Source: CAD feature listing. Evaluate the final solid. Frame: model axes, mm. Face numbers are marked on the shaded views. A direction names the side the tool comes from. Round coordinates to 2 decimals unless told otherwise and drop trailing zeros. Order: outer loops, then holes, each group sorted by start corner. A loop starts at its lowest first (then second) coordinate and runs counter-clockwise, first axis right, second up. Notation, with made-up numbers: (10.25, 52) - (53.25, 52) arc R8 ccw to (53.25, 62) - close; hole circle Ø1 at (-25.5, 9.25). An arc over 180 degrees is marked (long way). Use one line per item in the form item = value. Start each with the question number.
Q1. Ray query, line 1 (Y direction, x = 28, z = -6.5); line 2 (Y direction, x = 25.5, z = -3.75); line 3 (X direction, y = -16, z = -9). Return the intervals inside material, ascending. Write a range as [from, to].
Q2. Pin query (flat end, axial travel): pin 1 Ø1.5 at (x, z) = (26, -7) entering from +Y; pin 2 Ø4 at (x, z) = (-2.5, -6.5) entering from +Y; pin 3 Ø13.5 at (x, y) = (0, 0) entering from -Z. Return the tip coordinate at first contact, or that it passes through.
Q3. Cut plane C-C, the plane y = 19. Return the cut outline in (x, z), and give its area (3 significant figures).
Q4. Draft query along Y for the marked faces 5, 6, 7 and 8. Return one class per face: released by +Y, released by -Y, zero draft, split by the parting line, or undercut.
Q5. Set-up query: the marked faces 1, 2, 3 and 4. Return all of +Z, -Z, +X, -X, +Y, -Y with unobstructed straight access to the full face (end or side cutting, diameter ignored); none if empty.
Q6. Cut plane A-A, the plane y = 6. Return the cut outline in (x, z), and give its area (3 significant figures).
Q7. Cut plane B-B, the plane y = -3. Return the cut outline in (x, z), and give its area (3 significant figures).
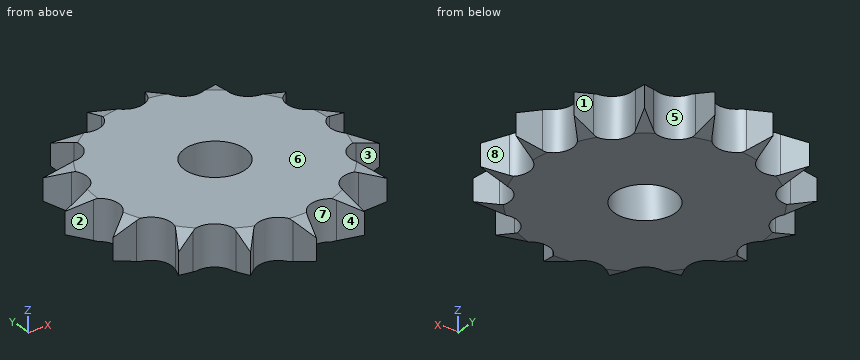
from build123d import *

# Parameters (mm, degrees)
IZIM1_R                     = 35
Y_KSEKLIK_EKSTR_ZYON1_DEPTH = 10
KES_EKSTR_ZYON1_DEPTH       = 10
DAIRESEL_KAPLAMA1_COUNT     = 15
IZIM8_R                     = 7.5
KES_EKSTR_ZYON2_DEPTH       = 10


with BuildPart() as part:
    # Çizim1 → Yükseklik-Ekstrüzyon1 (new body)
    with BuildSketch(Plane.XY):
        Circle(IZIM1_R)
    extrude(amount=-Y_KSEKLIK_EKSTR_ZYON1_DEPTH)

    # Çizim2 → Kes-Ekstrüzyon1 (cut)
    with BuildSketch(Plane.XY):
        with BuildLine():
            Line((-4.330127019, 29.061737365), (-9.008699853, 37.16526322))
            Line((-9.008699853, 37.16526322), (9.008699853, 37.16526322))
            Line((9.008699853, 37.16526322), (4.330127019, 29.061737365))
            ThreePointArc((4.330127019, 29.061737365), (0, 26.561737365), (-4.330127019, 29.061737365))
        make_face()
    kes_ekstr_zyon1 = extrude(amount=-KES_EKSTR_ZYON1_DEPTH, mode=Mode.SUBTRACT)

    # Dairesel Kaplama1: Kes-Ekstrüzyon1 ×15 about axis
    dairesel_kaplama1_axis = Axis((0, 0, 0), (0, 0, 1))
    for i in range(1, DAIRESEL_KAPLAMA1_COUNT):
        add(kes_ekstr_zyon1.rotate(dairesel_kaplama1_axis, i * 360 / DAIRESEL_KAPLAMA1_COUNT), mode=Mode.SUBTRACT)

    # Çizim8 → Kes-Ekstrüzyon2 (cut)
    with BuildSketch(Plane.XY):
        Circle(IZIM8_R)
    extrude(amount=-KES_EKSTR_ZYON2_DEPTH, mode=Mode.SUBTRACT)

    # Çizim11 → Kes-Döndür1 (revolve, cut)
    with BuildSketch(Plane(origin=(0, 0, 0), x_dir=(0, 0, -1), z_dir=(1, 0, 0))):
        Polygon((0, 28.561737365), (2.911761874, 36.561737365), (0, 36.561737365), align=None)
        Polygon((10, 36.561737365), (7.088238126, 36.561737365), (10, 28.561737365), align=None)
    revolve(axis=Axis((0, 0, 2.836239844), (0, 0, -1)), mode=Mode.SUBTRACT)


solid = part.part
Completed:
q1.line_1 = [-10.78, -6.98], [0.38, 5.18], [14.99, 16.97]
q1.line_2 = [-23.15, -22.61], [-11.13, 7.61], [11.9, 16.44]
q1.line_3 = [-22.34, 22.34]
q2.pin_1 = 16.71
q2.pin_2 = 29.36
q2.pin_3 = through
q3.outline = (-18.93, -10) - (18.93, -10) - (18.93, 0) - (-18.93, 0) - close
q3.area = 379 mm2
q4.face_5 = released by +Y
q4.face_6 = zero draft
q4.face_7 = released by -Y
q4.face_8 = undercut
q5.face_1 = +Z, -Z, +Y
q5.face_2 = +Z, -Z, -X
q5.face_3 = +Z, -Z, +X, -Y
q5.face_4 = +Z, -Z, -Y
q6.outline = (-26.71, -10) - (-4.5, -10) - (-4.5, 0) - (-26.71, 0) - close; (4.5, -10) - (26.71, -10) - (26.71, 0) - (4.5, 0) - close
q6.area = 444 mm2
q7.outline = (-26.4, -10) - (-6.87, -10) - (-6.87, 0) - (-26.4, 0) - close; (6.87, -10) - (26.4, -10) - (26.4, 0) - (6.87, 0) - close
q7.area = 390 mm2
